Geometry check sheet. Reference: the model listing, model coordinates, mm. Coordinates: 2 decimals unless noted, no trailing zeros. Loops run counter-clockwise (first coordinate to the right, second up) from the corner with the lowest first, then second, coordinate; pieces in that order, holes last.
from build123d import *

# Parameters (mm, degrees)
CROQUIS1_W              = 1250
CROQUIS1_H              = 1000
SALIENTE_EXTRUIR1_DEPTH = 17
CROQUIS2_W              = 75
CROQUIS2_H              = 75
SALIENTE_EXTRUIR2_DEPTH = 700


with BuildPart() as part:
    # Croquis1 → Saliente-Extruir1 (new body)
    with BuildSketch(Plane(origin=(0, 0, 0), x_dir=(1, 0, 0), z_dir=(0, 1, 0))):
        Rectangle(CROQUIS1_W, CROQUIS1_H)
    extrude(amount=SALIENTE_EXTRUIR1_DEPTH)

    # Croquis2 → Saliente-Extruir2 (add)
    with BuildSketch(Plane(origin=(0, 17, 0), x_dir=(1, 0, 0), z_dir=(0, 1, 0))):
        with Locations((-587.5, -462.5)):
            Rectangle(CROQUIS2_W, CROQUIS2_H)
        with Locations((-587.5, 462.5)):
            Rectangle(CROQUIS2_W, CROQUIS2_H)
        with Locations((587.5, -462.5)):
            Rectangle(CROQUIS2_W, CROQUIS2_H)
        with Locations((587.5, 462.5)):
            Rectangle(CROQUIS2_W, CROQUIS2_H)
    extrude(amount=-SALIENTE_EXTRUIR2_DEPTH)


solid = part.part
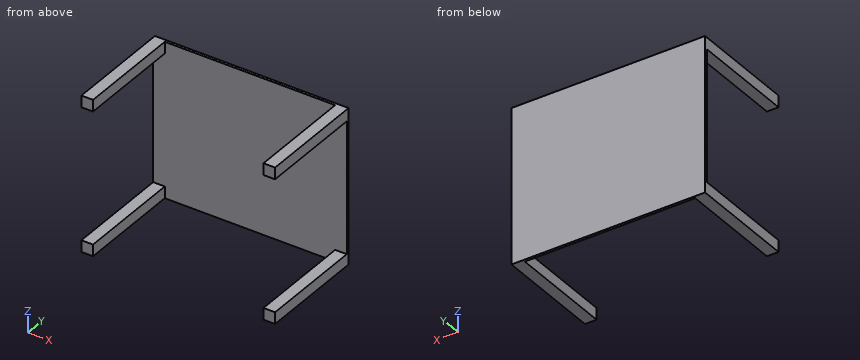
1) Section check A-A on y = -633.5. Record the cut outline in (x, z).
Data:
outline: (-625, -500) - (-550, -500) - (-550, -425) - (-625, -425) - close; (-625, 425) - (-550, 425) - (-550, 500) - (-625, 500) - close; (550, -500) - (625, -500) - (625, -425) - (550, -425) - close; (550, 425) - (625, 425) - (625, 500) - (550, 500) - close
2) Section check C-C on z = 7. Record the cut outline in (x, y), and give its area (4 significant figures).
Data:
outline: (-625, 0) - (625, 0) - (625, 17) - (-625, 17) - close
area: 21,250 mm2
3) Section check B-B on x = -338. Record the cut outline in (y, z).
Data:
outline: (0, -500) - (17, -500) - (17, 500) - (0, 500) - close
4) Depth check by flat-ended pin: pin 1 (12 mm diameter, centred on x = 104, z = -304, fed in from -Y). Enter the tip coordinate at first touch or a pass-through.
Data:
pin 1: stops at y = 0
5) Material ranges on probe 1 along Y at (x, z) = (535, 315.5), recorded low to high.
Data:
probe 1: y = 0 to 17
